```python
from build123d import *

# Parameters (mm, degrees)
F0_R     = 2.5
F1_DEPTH = 3
F2_R     = 2.5
F3_DEPTH = 1
F5_DEPTH = 1


with BuildPart() as f1:
    # F0 (on Top) → F1 (new body)
    with BuildSketch(Plane.XY):
        with BuildLine():
            Line((-10.03743, -4.5), (-10.03743, 4.5))
            ThreePointArc((-10.03743, 4.5), (-11, 0), (-10.03743, -4.5))
        make_face()
        with BuildLine():
            ThreePointArc((-6.78233, -3.75), (-7.75, 0), (-6.78233, 3.75))
            Line((-6.78233, 3.75), (-10.03743, 4.5))
            Line((-10.03743, 4.5), (-10.03743, -4.5))
            Line((-10.03743, -4.5), (-6.78233, -3.75))
        make_face()
        with BuildLine():
            ThreePointArc((-6.78233, 3.75), (1.93642, 7.504184), (7.75, 0))
            ThreePointArc((7.75, 0), (1.93642, -7.504184), (-6.78233, -3.75))
            Line((-6.78233, -3.75), (-10.03743, -4.5))
            ThreePointArc((-10.03743, -4.5), (-5.97913, -9.233093), (0, -11))
            Line((0, -11), (30, -11))
            ThreePointArc((30, -11), (41, 0), (30, 11))
            Line((30, 11), (0, 11))
            ThreePointArc((0, 11), (-5.97913, 9.233093), (-10.03743, 4.5))
            Line((-10.03743, 4.5), (-6.78233, 3.75))
        make_face()
        with Locations((35, 0)):
            Circle(F0_R, mode=Mode.SUBTRACT)
        with BuildLine():
            Line((-6.78233, -3.75), (-6.78233, 3.75))
            ThreePointArc((-6.78233, 3.75), (-7.75, 0), (-6.78233, -3.75))
        make_face()
        with BuildLine():
            ThreePointArc((-6.78233, -3.75), (1.93642, -7.504184), (7.75, 0))
            ThreePointArc((7.75, 0), (1.93642, 7.504184), (-6.78233, 3.75))
            Line((-6.78233, 3.75), (-6.78233, -3.75))
        make_face()
    extrude(amount=F1_DEPTH)

    # F2
    f2_edges = [f1.edges().sort_by_distance(p)[0] for p in [
        (-11, 0, 3),
    ]]
    fillet(f2_edges, radius=F2_R)

    # F0 (on Top) → F3 (cut)
    with BuildSketch(Plane.XY):
        with BuildLine():
            Line((-10.03743, -4.5), (-10.03743, 4.5))
            ThreePointArc((-10.03743, 4.5), (-11, 0), (-10.03743, -4.5))
        make_face()
        with BuildLine():
            ThreePointArc((-6.78233, -3.75), (-7.75, 0), (-6.78233, 3.75))
            Line((-6.78233, 3.75), (-10.03743, 4.5))
            Line((-10.03743, 4.5), (-10.03743, -4.5))
            Line((-10.03743, -4.5), (-6.78233, -3.75))
        make_face()
        with BuildLine():
            Line((-6.78233, -3.75), (-6.78233, 3.75))
            ThreePointArc((-6.78233, 3.75), (-7.75, 0), (-6.78233, -3.75))
        make_face()
        with BuildLine():
            ThreePointArc((-6.78233, -3.75), (1.93642, -7.504184), (7.75, 0))
            ThreePointArc((7.75, 0), (1.93642, 7.504184), (-6.78233, 3.75))
            Line((-6.78233, 3.75), (-6.78233, -3.75))
        make_face()
    extrude(amount=F3_DEPTH, mode=Mode.SUBTRACT)

    # F4 (on face) → F5 (cut)
    with BuildSketch(Plane.XY.offset(3)):
        with BuildLine():
            ThreePointArc((36.9, -2.939388), (31.5, 0), (36.9, 2.939388))
            ThreePointArc((36.9, 2.939388), (34.135492, 6.256813), (30, 7.5))
            Line((30, 7.5), (0, 7.5))
            ThreePointArc((0, 7.5), (-7.5, 0), (0, -7.5))
            Line((0, -7.5), (30, -7.5))
            ThreePointArc((30, -7.5), (34.135492, -6.256813), (36.9, -2.939388))
        make_face()
    extrude(amount=-F5_DEPTH, mode=Mode.SUBTRACT)


solid = f1.part
```
The model under review builds one solid part; all positions refer to its coordinate system, in mm. A direction names the side the tool comes from. Round coordinates to 2 decimals unless told otherwise and drop trailing zeros. Loops run counter-clockwise (first coordinate to the right, second up) from the corner with the lowest first, then second, coordinate; pieces in that order, holes last. Notation, with made-up numbers: M -38,57.25 L 7,57.25 A17 ccw 7,74.25 Z; hole C 17,-6.5 d11. An arc over 180 degrees is marked long. Answer as a JSON object with one key per item and string values.
(1) Tool access review of faces 1 (the flat face through (14.8, -7.5, 2.5)), 2 (the cylindrical face through (41, -0.2, 0.2)), 3 (the flat face through (-8.39, 4.12, 0.49)): name each direction out of +Z, -Z, +X, -X, +Y, -Y from which nothing blocks a thin tool from reaching the whole face with its end or side.
Resolved:
{"face 1": "+Z", "face 2": "+Z, -Z, +X", "face 3": "-Z, -X"}
(2) Take a section at A-A on x = 21. Give the boundary of the cut face in (y, z).
Resolved:
{"outline": "M -11,0 L 11,0 L 11,0.5 A2.5 ccw 8.5,3 L 7.5,3 L 7.5,2 L -7.5,2 L -7.5,3 L -8.5,3 A2.5 ccw -11,0.5 Z"}
(3) Take a section at C-C on x = 1. Give the boundary of the cut face in (y, z).
Resolved:
{"outline": "M -11,0 L -7.69,0 L -7.69,1 L 7.69,1 L 7.69,0 L 11,0 L 11,0.5 A2.5 ccw 8.5,3 L 7.5,3 L 7.5,2 L -7.5,2 L -7.5,3 L -8.5,3 A2.5 ccw -11,0.5 Z"}
(4) Draft analysis for pull direction X (two halves, no side actions). For faces 4 (the flat face through (21, 0, 0)), 5 (the flat face through (-8.43, -4.13, 0.49)), 6 (the flat face through (-2, 0, 1)), 7 (the flat face through (15.2, 7.5, 2.5)), state which applies: released by +X, released by -X, zero draft, split by the parting line, or undercut.
Resolved:
{"face 4": "zero draft", "face 5": "released by -X", "face 6": "undercut", "face 7": "undercut"}
(5) To check wall thickness, follow line 1 along Y through (x, z) = (35, 2.15); line 2 along X through (y, z) = (-1.75, 2.35); line 3 along Z through (x, y) = (22, 6). State the ranges of each line that lie inside material, in increasing order.
Resolved:
{"line 1": "-9.09 to -5.59, -3.5 to -2.5, 2.5 to 3.5, 5.59 to 9.09", "line 2": "-10.03 to -7.29, 31.97 to 33.21, 36.79 to 40.03", "line 3": "0 to 2"}
(6) Take a section at B-B on x = 7. Give the boundary of the cut face in (y, z), and give its area (3 significant figures).
Resolved:
{"outline": "M -11,0 L -3.33,0 L -3.33,1 L 3.33,1 L 3.33,0 L 11,0 L 11,0.5 A2.5 ccw 8.5,3 L 7.5,3 L 7.5,2 L -7.5,2 L -7.5,3 L -8.5,3 A2.5 ccw -11,0.5 Z", "area": "41.7 mm²"}
(7) Clearance check with flat-ended pins moving along their axes: P1, Ø3, axis at x = 35, y = 0, coming from the -Z side; P2, Ø4.5, axis at x = 2, y = -1.5, coming from the -Z side; P3, Ø1.1, axis at x = 21, z = 2.5, coming from the -Y side; P4, Ø6, axis at x = 10, y = -4, coming from the +Z side. State where each tip first meets the part, or that it passes through.
Resolved:
{"P1": "through", "P2": "z = 1", "P3": "y = -10.54", "P4": "z = 2"}
